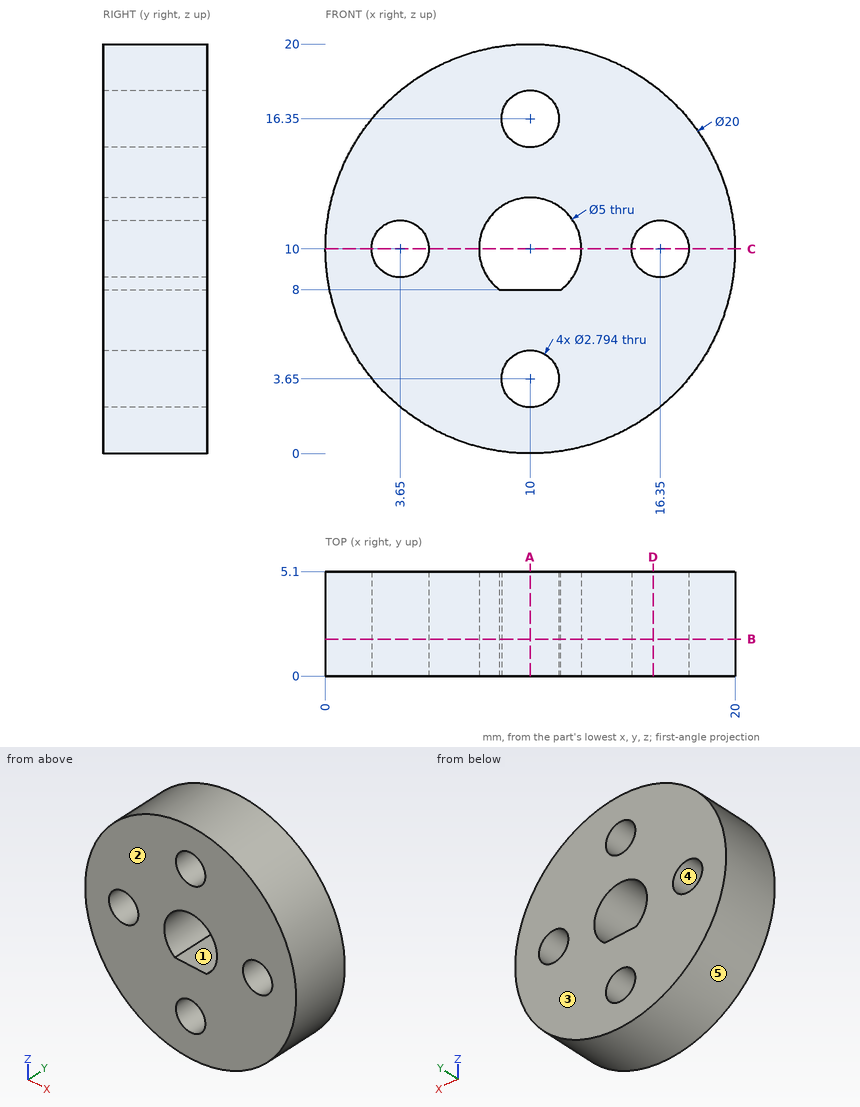
Check sheet for the drawn part. Datum: minimum x, y, z corner. Units: mm. A direction names the side the tool comes from. Round coordinates to 2 decimals unless told otherwise and drop trailing zeros. Order: outer loops, then holes, each group sorted by start corner. A loop starts at its lowest first (then second) coordinate and runs counter-clockwise, first axis right, second up. Notation, with made-up numbers: M 75.25,-14 L 84.25,-14 A17 ccw 84.25,-6 Z; hole C 57.25,-30.75 d2. An arc over 180 degrees is marked long. Write each question's results on one line, items separated by ' | '. Start each with the question number.
1. Cross-section at A-A on x = 10. Record the boundary of the cut face in (y, z), plus the area to 3 significant figures.
2. Draft check along Z on the marked faces 3, 4 and 5. Enter one of: pulls with the +Z half, pulls with the -Z half, needs draft (parallel to the pull), parting line crosses it, or undercut.
3. Set-up check for the marked faces 1 and 2: record each of +Z, -Z, +X, -X, +Y, -Y from which the full face is reachable in a straight line by a thin tool's end or side.
4. Material ranges on L1, parallel to X at y = 2.2, z = 10; L2, parallel to X at y = 0.35, z = 11; L3, parallel to Z at x = 10.25, y = 3.85, recorded low to high. Write a range as from..to.
5. Cross-section at B-B on y = 1.8. Record the boundary of the cut face in (x, z).
6. Cross-section at C-C on z = 10. Record the boundary of the cut face in (x, y).
7. Cross-section at D-D on x = 16. Record the boundary of the cut face in (y, z), plus the area to 3 significant figures.
8. Go/stop test with flat-tipped pins: P1, Ø1.5, axis at x = 3, z = 2.5, coming from the +Y side; P2, Ø1.5, axis at x = 16.5, y = 4, coming from the -Z side; P3, Ø2, axis at x = 16.5, y = 2, coming from the +Z side; P4, Ø3, axis at x = 17.5, y = 3.5, coming from the +Z side. Record where each tip stops, or that it passes through.
Resolved:
1) outline: M 0,0 L 5.1,0 L 5.1,2.25 L 0,2.25 Z; M 0,5.05 L 5.1,5.05 L 5.1,8 L 0,8 Z; M 0,12.5 L 5.1,12.5 L 5.1,14.95 L 0,14.95 Z; M 0,17.75 L 5.1,17.75 L 5.1,20 L 0,20 Z | area: 50.6 mm2
2) face 3: needs draft | face 4: undercut | face 5: parting line crosses it
3) face 1: +Y, -Y | face 2: +Z, -Z, +X, -X, -Y
4) L1: 0..2.25, 5.05..7.5, 12.5..14.95, 17.75..20 | L2: 0.05..2.67, 4.63..7.71, 12.29..15.37, 17.33..19.95 | L3: 0..2.28, 5.02..8, 12.49..14.98, 17.72..20
5) outline: C 10,10 d20; hole C 3.65,10 d2.79; hole M 8.5,8 L 11.5,8 A2.5 ccw long Z; hole C 10,3.65 d2.79; hole C 10,16.35 d2.79; hole C 16.35,10 d2.79
6) outline: M 0,0 L 2.25,0 L 2.25,5.1 L 0,5.1 Z; M 5.05,0 L 7.5,0 L 7.5,5.1 L 5.05,5.1 Z; M 12.5,0 L 14.95,0 L 14.95,5.1 L 12.5,5.1 Z; M 17.75,0 L 20,0 L 20,5.1 L 17.75,5.1 Z
7) outline: M 0,2 L 5.1,2 L 5.1,8.65 L 0,8.65 Z; M 0,11.35 L 5.1,11.35 L 5.1,18 L 0,18 Z | area: 67.8 mm2
8) P1: y = 5.1 | P2: z = 1.82 | P3: z = 18.35 | P4: z = 18
